from build123d import *

# Parameters (mm, degrees)
SKETCH1_W           = 7.25
SKETCH1_H           = 12.5
BOSS_EXTRUDE1_DEPTH = 5.4
SKETCH3_W           = 2.5
SKETCH3_H           = 3.5
SKETCH3_W_2         = 1
SKETCH3_H_2         = 0.331350256
BOSS_EXTRUDE2_DEPTH = 3


with BuildPart() as part:
    # Sketch1 → Boss-Extrude1 (new body)
    with BuildSketch(Plane.XY):
        with Locations((3.625, 6.25)):
            Rectangle(SKETCH1_W, SKETCH1_H)
    extrude(amount=BOSS_EXTRUDE1_DEPTH)

    # Sketch3 → Boss-Extrude2 (add)
    with BuildSketch(Plane(origin=(7.25, 0, 0), x_dir=(0, 0, -1), z_dir=(1, 0, 0))):
        with Locations((-2.7, 6.25)):
            Rectangle(SKETCH3_W, SKETCH3_H)
        with Locations((-2.303664878, 5.686580017)):
            Rectangle(SKETCH3_W_2, SKETCH3_H_2, mode=Mode.SUBTRACT)
        with Locations((-2.303664878, 6.813419983)):
            Rectangle(SKETCH3_W_2, SKETCH3_H_2, mode=Mode.SUBTRACT)
    extrude(amount=BOSS_EXTRUDE2_DEPTH)


solid = part.part
Design review of the part built by this model. Coordinates are the model's own, in mm. A direction names the side the tool comes from. Round coordinates to 2 decimals unless told otherwise and drop trailing zeros. Write each loop counter-clockwise with the first axis right and the second up, starting at its lowest first coordinate (ties: lowest second). Pieces come first, ordered by that corner, then holes.
Item 1: Draft analysis for pull direction Y (two halves, no side actions). For faces 6 (the flat face through (9, 6.648, 2)), 7 (the flat face through (4, 12.5, 3)), 8 (the flat face through (9, 6, 3.95)), state which applies: released by +Y, released by -Y, zero draft, split by the parting line, or undercut.
Item 2: Consider section D-D on y = 9.5. Give the boundary of the cut face in (x, z).
Item 3: Consider section B-B on z = 3. Give the boundary of the cut face in (x, y), and give its area (3 significant figures).
Item 4: For pin 1 Ø1 at (x, z) = (9, 1.5) entering from -Y; pin 2 Ø1.5 at (x, y) = (9.5, 5.5) entering from +Z; pin 3 Ø0.5 at (x, z) = (8.5, 2.5) entering from +Y, all flat-tipped, find the tip position at first contact; note any pin that passes through.
Item 5: Wall thickness on L1, parallel to X at y = 10, z = 3.7; L2, parallel to Y at x = 8.5, z = 1.6: over which ranges is each line inside the solid? List them lowest first.
Item 6: Consider section C-C on y = 7.5. Give the boundary of the cut face in (x, z), and give its area (4 significant figures).
Item 7: For faces 1 (the flat face through (9, 4.5, 3)), 2 (the flat face through (9, 5.521, 2)), 3 (the flat face through (9, 6, 1.45)), 4 (the flat face through (9, 8, 3)), 5 (the flat face through (4, 0, 3)), list the 3-axis set-ups (+Z, -Z, +X, -X, +Y, -Y) from which the entire face can be reached by the end or side of a thin tool; tool diameter is ignored.
Item 8: Consider section A-A on x = 8. Give the boundary of the cut face in (y, z), and give its area (3 significant figures).
Check values:
1. face 6: undercut
1. face 7: released by +Y
1. face 8: zero draft
2. outline: (0, 0) - (7.25, 0) - (7.25, 5.4) - (0, 5.4) - close
3. outline: (0, 0) - (7.25, 0) - (7.25, 4.5) - (10.25, 4.5) - (10.25, 8) - (7.25, 8) - (7.25, 12.5) - (0, 12.5) - close
3. area: 101 mm2
4. pin 1: stops at y = 4.5
4. pin 2: stops at z = 3.95
4. pin 3: stops at y = 8
5. L1: x = 0 to 7.25
5. L2: y = 4.5 to 8
6. outline: (0, 0) - (7.25, 0) - (7.25, 1.45) - (10.25, 1.45) - (10.25, 3.95) - (7.25, 3.95) - (7.25, 5.4) - (0, 5.4) - close
6. area: 46.65 mm2
7. face 1: +Z, -Z, +X, -Y
7. face 2: +X
7. face 3: -Z, +X, +Y, -Y
7. face 4: +Z, -Z, +X, +Y
7. face 5: +Z, -Z, +X, -X, -Y
8. outline: (4.5, 1.45) - (8, 1.45) - (8, 3.95) - (4.5, 3.95) - close; hole (5.52, 1.8) - (5.85, 1.8) - (5.85, 2.8) - (5.52, 2.8) - close; hole (6.65, 1.8) - (6.98, 1.8) - (6.98, 2.8) - (6.65, 2.8) - close
8. area: 8.09 mm2
